Input: part model. Units: mm. Frame: model coordinates. Face numbers are marked on the shaded views. Round coordinates to 2 decimals unless told otherwise and drop trailing zeros. Loops run counter-clockwise (first coordinate to the right, second up) from the corner with the lowest first, then second, coordinate; pieces in that order, holes last. Notation, with made-up numbers: M 50.25,19 L 104.25,19 A34 cw 104.25,52 Z; hole C 10.5,-38 d6. An arc over 180 degrees is marked long. Return JSON: item names as keys, results as strings. Group by question number.
1) Section B-B (x = 20). Output: boundary loops of the cut face in (y, z).
2) Material intervals for line 1 (Y direction, x = 0, z = 4.3); line 2 (X direction, y = 17.5, z = 4.3); line 3 (X direction, y = -5, z = 4.4), sorted ascending. Write a range as from..to.
3) Section D-D (y = -15). Output: boundary loops of the cut face in (x, z).
4) Section C-C (z = 4.2). Output: boundary loops of the cut face in (x, y).
5) Contact query for flat-ended pins moving along their axis: P1, Ø1.8, axis at x = 10, y = 17.32, coming from the +Z side; P2, Ø1.5, axis at y = -1, z = 5, coming from the +X side. Output: stop coordinate, or through.
6) Mould query, pull axis Y, two halves, no side actions, for the marked faces 1, 2 and 3. Classes: +Y half, -Y half, draft (parallel to the pull), parting line (faces both ways), or undercut.
7) Section A-A (y = 0). Output: boundary loops of the cut face in (x, z).
from build123d import *

# Parameters (mm, degrees)
CYLINDER_R      = 25
CYLINDER_DEPTH  = 4
SKETCH_R        = 1.5
POCKET_DEPTH    = 4.001
SKETCH001_R     = 10
POCKET001_DEPTH = 5


with BuildPart() as part:
    # Cylinder → Cylinder (new body)
    with BuildSketch(Plane.XY.offset(2)):
        Circle(CYLINDER_R)
    extrude(amount=CYLINDER_DEPTH)

    # Sketch → Pocket (cut, through all)
    with BuildSketch(Plane.XY.offset(6)):
        with Locations((20, 0)):
            Circle(SKETCH_R)
        with Locations((-10, 17.320508)):
            Circle(SKETCH_R)
        with Locations((-10, -17.320508)):
            Circle(SKETCH_R)
        with Locations((-20, 0)):
            Circle(SKETCH_R)
        with Locations((10, -17.320508)):
            Circle(SKETCH_R)
        with Locations((10, 17.320508)):
            Circle(SKETCH_R)
    extrude(amount=-POCKET_DEPTH, mode=Mode.SUBTRACT)

    # Sketch001 → Pocket001 (cut)
    with BuildSketch(Plane.XY.offset(6)):
        Circle(SKETCH001_R)
    extrude(amount=-POCKET001_DEPTH, mode=Mode.SUBTRACT)


solid = part.part
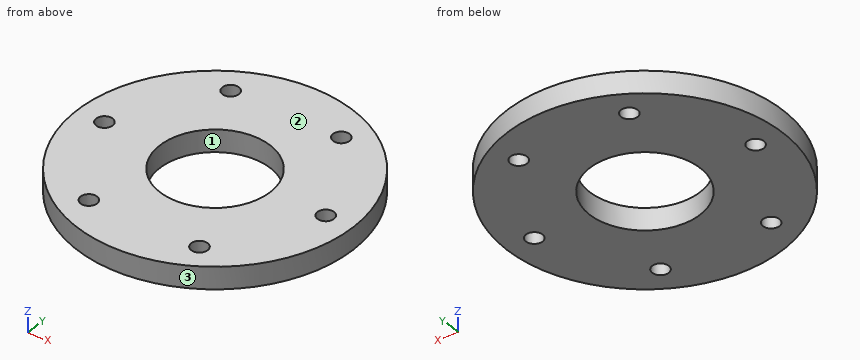
Returned:
{
 "1": {"outline": "M -15,2 L -1.5,2 L -1.5,6 L -15,6 Z; M 1.5,2 L 15,2 L 15,6 L 1.5,6 Z"},
 "2": {"line 1": "y = -25..-10, 10..25", "line 2": "x = -17.85..-11.49, -8.51..8.51, 11.49..17.85", "line 3": "x = -24.49..-8.66, 8.66..24.49"},
 "3": {"outline": "M -20,2 L 20,2 L 20,6 L -20,6 Z"},
 "4": {"outline": "C 0,0 d50; hole C -20,0 d3; hole C -10,-17.32 d3; hole C -10,17.32 d3; hole C 0,0 d20; hole C 10,-17.32 d3; hole C 10,17.32 d3; hole C 20,0 d3"},
 "5": {"P1": "passes through", "P2": "stops at x = 25"},
 "6": {"face 1": "undercut", "face 2": "draft", "face 3": "parting line"},
 "7": {"outline": "M -25,2 L -21.5,2 L -21.5,6 L -25,6 Z; M -18.5,2 L -10,2 L -10,6 L -18.5,6 Z; M 10,2 L 18.5,2 L 18.5,6 L 10,6 Z; M 21.5,2 L 25,2 L 25,6 L 21.5,6 Z"}
}
